Geometry check sheet. Reference: the model listing, model coordinates, mm. Face numbers are marked on the shaded views. A direction names the side the tool comes from. Coordinates: 2 decimals unless noted, no trailing zeros. Loops run counter-clockwise (first coordinate to the right, second up) from the corner with the lowest first, then second, coordinate; pieces in that order, holes last. Notation, with made-up numbers: M 42.25,-13 L 48.25,-13 A13 cw 48.25,10 Z; hole C 35,-15 d4. An arc over 180 degrees is marked long. Use CSV: the item, a comma, the result in double quotes.
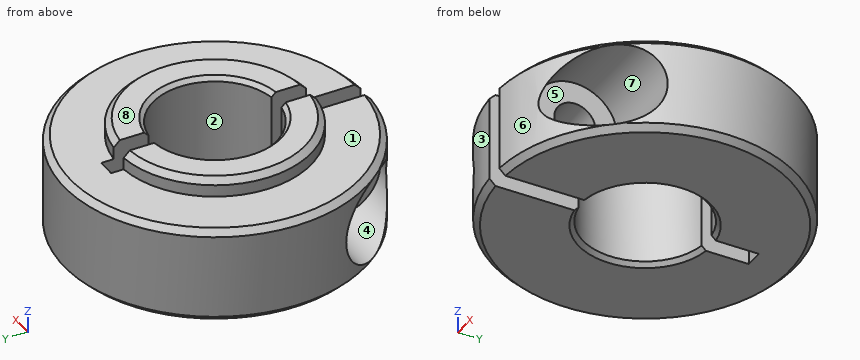
Autodesk Inventor part; units mm, degrees
ref_plane "body_screw_XY" through (4, -8, 0) normal (1, 0, 0) x (0, 0, -1)
ref_plane "body_screw_YZ" through (4, -8, 0) normal (0, 0, -1) x (0, 1, 0)
ref_plane "body_screw_ZX" through (4, -8, 0) normal (0, 1, 0) x (1, 0, 0)
sketch "Sketch_1" plane through (0, 0, 0) normal (1, 0, 0) x (0, 1, 0)
  line L0 (0, -4) -> (0, 5.5)
  line L1 (7.5, 5.5) -> (5.5, 5.5)
  line L2 (5.5, 5.5) -> (5, 5)
  line L3 (5, 5) -> (5, -3.5)
  line L4 (5, -3.5) -> (5.5, -4)
  line L5 (5.5, -4) -> (12, -4)
  line L6 (12, -4) -> (12.5, -3.5)
  line L7 (12.5, -3.5) -> (12.5, 3.5)
  line L8 (12.5, 3.5) -> (12, 4)
  line L9 (12, 4) -> (8, 4)
  line L10 (8, 4) -> (8, 5)
  line L11 (8, 5) -> (7.5, 5.5)
revolve "Revolution1" add sketch "Sketch_1" angle 360 about axis through (0, 0, -4) along (0, 0, -1)
sketch "Sketch_2" plane through (0, 0, 0) normal (0, 0, 1) x (1, 0, 0)
  line L0 (-0.75, -12.5) -> (0.75, -12.5)
  line L1 (0.75, -12.5) -> (0.75, 9)
  line L2 (0.75, 9) -> (-0.75, 9)
  line L3 (-0.75, 9) -> (-0.75, -12.5)
extrude "Extrusion1" cut sketch "Sketch_2" along normal mid plane 32
sketch "Sketch_3" plane through (0, 0, 0) normal (0, 0, 1) x (1, 0, 0)
  line L0 (0, -8) -> (12.5, -8)
  line L1 (12.5, -8) -> (12.5, -11)
  line L2 (12.5, -11) -> (4, -11)
  line L3 (4, -11) -> (4, -9.75)
  line L4 (4, -9.75) -> (0, -9.75)
  line L5 (0, -9.75) -> (0, -8)
  line L6 (0, -8) -> (12.5, -8)
ref_plane "body_screw_XY" through (4, -8, 0) normal (1, 0, 0) x (0, 0, -1)
ref_plane "body_screw_YZ" through (4, -8, 0) normal (0, 0, -1) x (0, 1, 0)
ref_plane "body_screw_ZX" through (4, -8, 0) normal (0, 1, 0) x (1, 0, 0)
ref_plane "作業平面5" through (4, -8, 0) normal (1, 0, 0) x (0, 0, -1)
sketch "スケッチ5" plane through (4, -8, 0) normal (1, 0, 0) x (0, 0, -1)
  point P0 (0, 8)
ref_plane "作業平面6" through (4, -8, 0) normal (1, 0, 0) x (0, 0, -1)
sketch "スケッチ6" plane through (4, -8, 0) normal (1, 0, 0) x (0, 0, -1)
  point P0 (0, 8)
sketch "スケッチ7" plane through (0, 0, -4) normal (0, 0, -1) x (-1, 0, 0)
  circle A0 centre (0, 0) radius 5.15
  dimension "d12" = 10.3
extrude "押し出し2" cut sketch "スケッチ7" against normal blind 10
ref_plane "作業平面4" through (12.5, 0, 0) normal (1, 0, 0) x (0, 1, 0)
sketch "スケッチ8" plane through (12.5, 0, 0) normal (1, 0, 0) x (0, 1, 0)
  circle A0 centre (-8, 0) radius 1.75
  circle A1 centre (-8, 0) radius 1.7
  circle A2 centre (-8, 0) radius 3.5
  point P0 (0, 0)
  dimension "d15" = 3.4
  dimension "d16" = 7
extrude "押し出し3" cut sketch "スケッチ8" against normal through all contours A1
extrude "押し出し4" cut sketch "スケッチ8" against normal blind 8.5 contours A0 | A1 | A2
mirror "ミラー1" about plane through (0, 0, 0) normal (1, 0, 0) of "押し出し4"
properties part number "SCBNJ10-16b" material "ABS プラスチック"
1. Set-up check for the marked faces 1, 2, 3, 4 and 5: record each of +Z, -Z, +X, -X, +Y, -Y from which the full face is reachable in a straight line by a thin tool's end or side.
The answers:
face 1,"+Z"
face 2,"+Z, -Z"
face 3,"+Z, -Z, -X, -Y"
face 4,"-X"
face 5,"+X"
2. Thickness scan on line 1 (Z direction, x = -6, y = -8); line 2 (X direction, y = -10, z = 3.25); line 3 (X direction, y = 8, z = 0.75). Record the ranges inside material, lowest first. Write a range as [from, to].
The answers:
line 1,"[-4, -3.5], [3.5, 4]"
line 2,"[-7.5, -0.75], [0.75, 7.5]"
line 3,"[-9.6, -0.75], [0.75, 9.6]"
3. Section check A-A, the plane y = 0. Record the cut outline in (x, z).
The answers:
outline,"M -12.5,-3.5 L -12,-4 L -5.5,-4 L -5.15,-3.65 L -5.15,5.15 L -5.5,5.5 L -7.5,5.5 L -8,5 L -8,4 L -12,4 L -12.5,3.5 Z; M 5.15,-3.65 L 5.5,-4 L 12,-4 L 12.5,-3.5 L 12.5,3.5 L 12,4 L 8,4 L 8,5 L 7.5,5.5 L 5.5,5.5 L 5.15,5.15 Z"
4. Gauge pin test, flat ends, axial feed: P1, Ø0.8, axis at x = 0, z = 1.5, coming from the -Y side; P2, Ø3, axis at y = 7.5, z = 0.5, coming from the -X side; P3, Ø1, axis at y = -4, z = 1.5, coming from the -X side; P4, Ø3, axis at x = -1, z = -0.5, coming from the -Y side. Record the tip position at first contact, or that the pin passes through.
The answers:
P1,"y = 9"
P2,"x = -10.97"
P3,"x = -12"
P4,"y = -12.48"
5. Section check B-B, the plane x = 0. Record the cut outline in (y, z), plus the area to 4 significant figures.
The answers:
outline,"M 9,-4 L 12,-4 L 12.5,-3.5 L 12.5,3.5 L 12,4 L 9,4 Z"
area,"27.75 mm^2"
6. Release check for a two-part mould opening along Y. For the marked faces 6, 7 and 8 record: +Y half, -Y half, draft (parallel to the pull), parting line (faces both ways), or undercut.
The answers:
face 6,"-Y half"
face 7,"undercut"
face 8,"draft"
7. Section check D-D, the plane z = 2.5. Record the cut outline in (x, y).
The answers:
outline,"M -11.2,-5.55 L -4,-5.55 L -4,-10.45 L -6.86,-10.45 A12.5 ccw -0.75,-12.48 L -0.75,-5.1 A5.15 cw -0.75,5.1 L -0.75,9 L 0.75,9 L 0.75,5.1 A5.15 cw 0.75,-5.1 L 0.75,-12.48 A12.5 ccw 6.86,-10.45 L 4,-10.45 L 4,-5.55 L 11.2,-5.55 A12.5 ccw long Z"
8. Section check C-C, the plane z = 0. Record the cut outline in (x, y).
The answers:
outline,"M -11.66,-4.5 L -4,-4.5 L -4,-6.3 L -0.75,-6.3 L -0.75,-5.1 A5.15 cw -0.75,5.1 L -0.75,9 L 0.75,9 L 0.75,5.1 A5.15 cw 0.75,-5.1 L 0.75,-6.3 L 4,-6.3 L 4,-4.5 L 11.66,-4.5 A12.5 ccw long Z; M -4.9,-11.5 A12.5 ccw -0.75,-12.48 L -0.75,-9.7 L -4,-9.7 L -4,-11.5 Z; M 0.75,-12.48 A12.5 ccw 4.9,-11.5 L 4,-11.5 L 4,-9.7 L 0.75,-9.7 Z"
